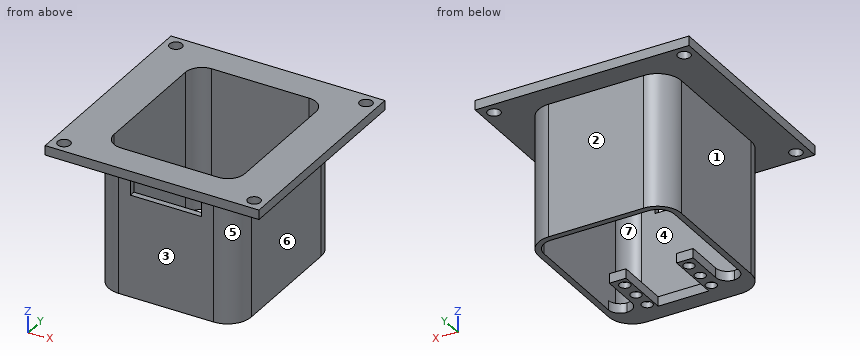
from build123d import *

# Parameters (mm, degrees)
SKETCH1_W           = 60
SKETCH1_H           = 70
BOSS_EXTRUDE1_DEPTH = 60
SKETCH2_R           = 1.25
BOSS_EXTRUDE2_DEPTH = 4
SKETCH4_W           = 30
SKETCH4_H           = 17
CUT_EXTRUDE1_DEPTH  = 2.5
SKETCH5_R           = 2.25
CUT_EXTRUDE2_DEPTH  = 2.5
SKETCH6_W           = 90
SKETCH6_H           = 90
SKETCH6_R           = 2.65
BOSS_EXTRUDE3_DEPTH = 4
FILLET1_R           = 10
CUT_EXTRUDE5_DEPTH  = 85.77027781
FILLET3_R           = 5
FILLET4_R           = 5


with BuildPart() as part:
    # Sketch1 → Boss-Extrude1 (new body)
    with BuildSketch(Plane.XY):
        Rectangle(SKETCH1_W, SKETCH1_H)
        with BuildLine():
            Line((20.5, -32.5), (-20.5, -32.5))
            ThreePointArc((-20.5, -32.5), (-25.449747468, -30.449747468), (-27.5, -25.5))
            Line((-27.5, -25.5), (-27.5, 25.5))
            ThreePointArc((-27.5, 25.5), (-25.449747468, 30.449747468), (-20.5, 32.5))
            Line((-20.5, 32.5), (20.5, 32.5))
            ThreePointArc((20.5, 32.5), (25.449747468, 30.449747468), (27.5, 25.5))
            Line((27.5, 25.5), (27.5, -25.5))
            ThreePointArc((27.5, -25.5), (25.449747468, -30.449747468), (20.5, -32.5))
        make_face(mode=Mode.SUBTRACT)
    extrude(amount=BOSS_EXTRUDE1_DEPTH)

    # Sketch2 → Boss-Extrude2 (add)
    with BuildSketch(Plane(origin=(0, 0, 0), x_dir=(-1, 0, 0), z_dir=(0, 0, -1))):
        with BuildLine():
            Line((-17.65, -4.5), (-10.65, -4.5))
            Line((-10.65, -4.5), (-10.65, -27.5))
            Line((-10.65, -27.5), (10.65, -27.5))
            Line((10.65, -27.5), (10.65, -4.5))
            Line((10.65, -4.5), (17.65, -4.5))
            Line((17.65, -4.5), (17.65, -25.5))
            Line((17.65, -25.5), (27.5, -25.5))
            ThreePointArc((27.5, -25.5), (25.449747468, -30.449747468), (20.5, -32.5))
            Line((20.5, -32.5), (-20.5, -32.5))
            ThreePointArc((-20.5, -32.5), (-25.449747468, -30.449747468), (-27.5, -25.5))
            Line((-27.5, -25.5), (-17.65, -25.5))
            Line((-17.65, -25.5), (-17.65, -4.5))
        make_face()
        with Locations((13.5, -8.5)):
            Circle(SKETCH2_R, mode=Mode.SUBTRACT)
        with Locations((13.5, -16.5)):
            Circle(SKETCH2_R, mode=Mode.SUBTRACT)
        with Locations((13.5, -24.5)):
            Circle(SKETCH2_R, mode=Mode.SUBTRACT)
        with Locations(Location((-13.5, -8.5, 0), (0, 0, 180))):
            Circle(SKETCH2_R, mode=Mode.SUBTRACT)
        with Locations(Location((-13.5, -16.5, 0), (0, 0, 180))):
            Circle(SKETCH2_R, mode=Mode.SUBTRACT)
        with Locations(Location((-13.5, -24.5, 0), (0, 0, 180))):
            Circle(SKETCH2_R, mode=Mode.SUBTRACT)
    extrude(amount=-BOSS_EXTRUDE2_DEPTH)

    # Sketch4 → Cut-Extrude1 (cut)
    with BuildSketch(Plane.XZ.offset(35)):
        with Locations((0, 51.5)):
            Rectangle(SKETCH4_W, SKETCH4_H)
    extrude(amount=-CUT_EXTRUDE1_DEPTH, mode=Mode.SUBTRACT)

    # Sketch5 → Cut-Extrude2 (cut)
    with BuildSketch(Plane(origin=(0, 0, 0), x_dir=(-1, 0, 0), z_dir=(0, 0, -1))):
        with Locations((-13.5, -8.5)):
            Circle(SKETCH5_R)
        with Locations((-13.5, -16.5)):
            Circle(SKETCH5_R)
        with Locations((-13.5, -24.5)):
            Circle(SKETCH5_R)
        with Locations((13.5, -24.5)):
            Circle(SKETCH5_R)
        with Locations((13.5, -16.5)):
            Circle(SKETCH5_R)
        with Locations((13.5, -8.5)):
            Circle(SKETCH5_R)
    extrude(amount=-CUT_EXTRUDE2_DEPTH, mode=Mode.SUBTRACT)

    # Sketch6 → Boss-Extrude3 (add)
    with BuildSketch(Plane.XY.offset(60)):
        Rectangle(SKETCH6_W, SKETCH6_H)
        with Locations((40, 40)):
            Circle(SKETCH6_R, mode=Mode.SUBTRACT)
        with Locations((-40, 40)):
            Circle(SKETCH6_R, mode=Mode.SUBTRACT)
        with Locations((-40, -40)):
            Circle(SKETCH6_R, mode=Mode.SUBTRACT)
        with Locations((40, -40)):
            Circle(SKETCH6_R, mode=Mode.SUBTRACT)
    extrude(amount=-BOSS_EXTRUDE3_DEPTH)

    # Fillet1
    fillet1_edges = [part.edges().sort_by_distance(p)[0] for p in [
        (-30, -35, 28),
        (30, -35, 28),
        (-30, 35, 28),
        (30, 35, 28),
    ]]
    fillet(fillet1_edges, radius=FILLET1_R)

    # Sketch8 → Cut-Extrude5 (cut, through all)
    with BuildSketch(Plane(origin=(0, 0, 56), x_dir=(-1, 0, 0), z_dir=(0, 0, -1))):
        with BuildLine():
            Line((-20.5, 32.5), (20.5, 32.5))
            ThreePointArc((20.5, 32.5), (25.449747468, 30.449747468), (27.5, 25.5))
            Line((27.5, 25.5), (27.5, -25.5))
            ThreePointArc((27.5, -25.5), (25.449747468, -30.449747468), (20.5, -32.5))
            Line((20.5, -32.5), (-20.5, -32.5))
            ThreePointArc((-20.5, -32.5), (-25.449747468, -30.449747468), (-27.5, -25.5))
            Line((-27.5, -25.5), (-27.5, 25.5))
            ThreePointArc((-27.5, 25.5), (-25.449747468, 30.449747468), (-20.5, 32.5))
        make_face()
    extrude(amount=-CUT_EXTRUDE5_DEPTH, mode=Mode.SUBTRACT)

    # Fillet3
    fillet3_edges = [part.edges().sort_by_distance(p)[0] for p in [
        (17.65, -25.5, 2),
        (-17.65, -25.5, 2),
    ]]
    fillet(fillet3_edges, radius=FILLET3_R)

    # Fillet4
    # the kernel refuses this fillet: 5 mm, written as the material it adds along each edge
    with BuildSketch(Plane(origin=(-27.5, -25.5, 0), x_dir=(1, 0, 0), z_dir=(0, 0, 1))) as fillet4_piece_1:
        with BuildLine():
            CenterArc((5, 4.997749494), FILLET4_R, 180, 88.280868679)
            Line((0, 4.997749494), (-0.1, 4.997749494))
            Line((-0.1, 4.997749494), (-0.1, 0))
            Line((-0.1, 0), (0, -0.1))
            ThreePointArc((0, -0.1), (2.425, -0.1), (4.847, -0.09995499))
            Line((4.847, -0.09995499), (4.85, 0))
        make_face()
    extrude(amount=4)
    with BuildSketch(Plane(origin=(27.5, -25.5, 0), x_dir=(0, 1, 0), z_dir=(0, 0, 1))) as fillet4_piece_2:
        with BuildLine():
            CenterArc((4.997749494, 5), FILLET4_R, 181.719131321, 88.280868679)
            Line((0, 4.85), (-0.09995499, 4.847))
            ThreePointArc((-0.09995499, 4.847), (-0.1, 2.425), (-0.1, 0))
            Line((-0.1, 0), (0, -0.1))
            Line((0, -0.1), (4.997749494, -0.1))
            Line((4.997749494, -0.1), (4.997749494, 0))
        make_face()
    extrude(amount=4)


solid = part.part
Can you work these out from the model? Positions are in its coordinate system, mm. Face numbers are marked on the shaded views. A direction names the side the tool comes from. Give positions to 0.01 mm unless a question says otherwise; leave off trailing zeros. Loops run counter-clockwise (first coordinate to the right, second up) from the corner with the lowest first, then second, coordinate; pieces in that order, holes last. Notation, with made-up numbers: (75, -2.75) - (92, -2.75) arc R28 ccw to (92, 33.25) - close; hole circle Ø3 at (-25, -28). An arc over 180 degrees is marked (long way). Answer as a JSON object with one key per item and string values.
Q1. Imagine slicing it at C-C on z = 40. Write out the boundary of the cut face in (x, y).
Geometry says:
{"outline": "(-30, -25) arc R10 ccw to (-20, -35) - (20, -35) arc R10 ccw to (30, -25) - (30, 25) arc R10 ccw to (20, 35) - (-20, 35) arc R10 ccw to (-30, 25) - close; hole (-27.5, -25.5) arc R7 ccw to (-20.5, -32.5) - (20.5, -32.5) arc R7 ccw to (27.5, -25.5) - (27.5, 25.5) arc R7 ccw to (20.5, 32.5) - (-20.5, 32.5) arc R7 ccw to (-27.5, 25.5) - close"}
Q2. Which directions (+Z, -Z, +X, -X, +Y, -Y) give clear straight access to the entire face, cutting with the end or side of a thin tool? Please do the marked faces 5, 6 and 7.
Geometry says:
{"face 5": "-Z, +X, -Y", "face 6": "-Z, +X, +Y, -Y", "face 7": "+Z"}
Q3. If I drill on L1, parallel to Y at x = -40, z = 58.45; L2, parallel to Y at x = -13.5, z = 0.5; L3, parallel to Y at x = 6, z = 41, over which ranges is the centre line in solid material (lowest first)?
Geometry says:
{"L1": "-45 to -42.65, -37.35 to 37.35, 42.65 to 45", "L2": "-35 to -26.75, -22.25 to -18.75, -14.25 to -10.75, -6.25 to -4.5, 32.5 to 35", "L3": "-35 to -32.5, 32.5 to 35"}
Q4. Imagine slicing it at B-B on y = 4.5. Write out the boundary of the cut face in (x, z).
Geometry says:
{"outline": "(-45, 56) - (-30, 56) - (-30, 0) - (-27.5, 0) - (-27.5, 60) - (-45, 60) - close; (27.5, 0) - (30, 0) - (30, 56) - (45, 56) - (45, 60) - (27.5, 60) - close"}
Q5. Imagine slicing it at A-A on x = -1. Write out the boundary of the cut face in (y, z).
Geometry says:
{"outline": "(-45, 56) - (-32.5, 56) - (-32.5, 60) - (-45, 60) - close; (-35, 0) - (-27.5, 0) - (-27.5, 4) - (-32.5, 4) - (-32.5, 43) - (-35, 43) - close; (32.5, 0) - (35, 0) - (35, 56) - (45, 56) - (45, 60) - (32.5, 60) - close"}
Q6. Imagine slicing it at D-D on z = 54.5. Write out the boundary of the cut face in (x, y), plus the area to 3 significant figures.
Geometry says:
{"outline": "(-30, -25) arc R10 ccw to (-20, -35) - (-15, -35) - (-15, -32.5) - (-20.5, -32.5) arc R7 cw to (-27.5, -25.5) - (-27.5, 25.5) arc R7 cw to (-20.5, 32.5) - (20.5, 32.5) arc R7 cw to (27.5, 25.5) - (27.5, -25.5) arc R7 cw to (20.5, -32.5) - (15, -32.5) - (15, -35) - (20, -35) arc R10 ccw to (30, -25) - (30, 25) arc R10 ccw to (20, 35) - (-20, 35) arc R10 ccw to (-30, 25) - close", "area": "506 mm²"}
Q7. If we mould it in two halves opening along Y, with no side actions, what happens to the marked faces 1, 2, 3 and 4? For each: pulls with the +Y half, pulls with the -Y half, needs draft (parallel to the pull), parting line crosses it, or undercut.
Geometry says:
{"face 1": "needs draft", "face 2": "pulls with the +Y half", "face 3": "pulls with the -Y half", "face 4": "undercut"}
Q8. Will these pins go through, and if not, where does the flat tip stop? P1, Ø10, axis at x = 10.5, z = 26.5, coming from the -Y side; P2, Ø4.5, axis at x = 13.5, z = 2, coming from the +Y side; P3, Ø10, axis at x = 18.5, y = -8, coming from the +Z side.
Geometry says:
{"P1": "y = -35", "P2": "y = 35", "P3": "z = 4"}
